Input: dimensioned drawing with shaded views. Units: mm. Origin: part minimum x, y, z. Give positions to 0.01 mm unless a question says otherwise; leave off trailing zeros. Loops run counter-clockwise (first coordinate to the right, second up) from the corner with the lowest first, then second, coordinate; pieces in that order, holes last.
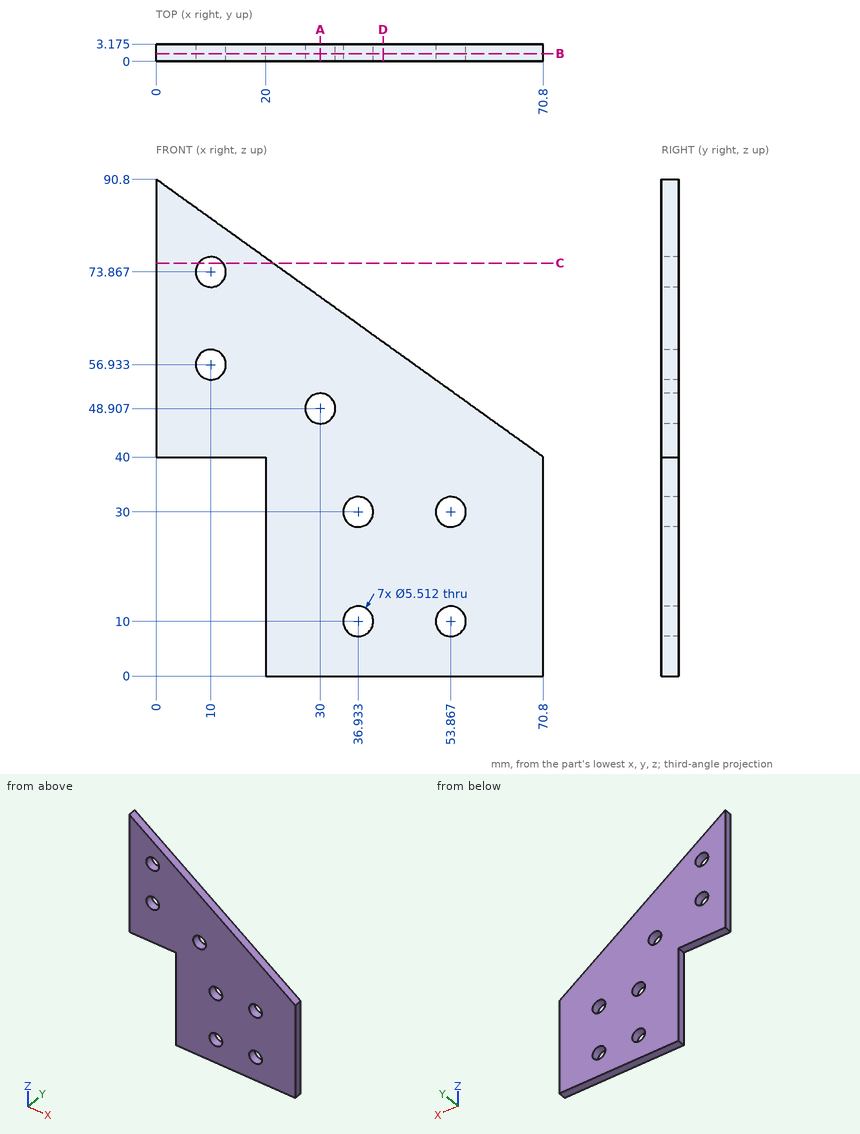
(1) Section A-A, the plane x = 30. Return the cut outline in (y, z) (1 decimal).
A:
outline: (0, 0) - (3.2, 0) - (3.2, 46.2) - (0, 46.2) - close; (0, 51.7) - (3.2, 51.7) - (3.2, 69.3) - (0, 69.3) - close
(2) Section B-B, the plane y = 1.4. Return the cut outline in (x, z), then the cut area to 3 significant figures.
A:
outline: (0, 40) - (20, 40) - (20, 0) - (70.8, 0) - (70.8, 40) - (0, 90.8) - close; hole circle Ø5.51 at (10, 56.93); hole circle Ø5.51 at (10, 73.87); hole circle Ø5.51 at (30, 48.91); hole circle Ø5.51 at (36.93, 10); hole circle Ø5.51 at (36.93, 30); hole circle Ø5.51 at (53.87, 10); hole circle Ø5.51 at (53.87, 30)
area: 3,660 mm2
(3) Section C-C, the plane z = 75.5. Return the cut outline in (x, y) (1 decimal).
A:
outline: (0, 0) - (7.8, 0) - (7.8, 3.2) - (0, 3.2) - close; (12.2, 0) - (21.3, 0) - (21.3, 3.2) - (12.2, 3.2) - close
(4) Ray query, line 1 along Z through (x, y) = (10, 2.7) (1 decimal); line 2 along X through (y, z) = (2, 28) (1 decimal); line 3 along Z through (x, y) = (34.5, 1.5) (1 decimal). Return the intervals inside material, ascending.
A:
line 1: z = 40 to 54.2, 59.7 to 71.1, 76.6 to 83.6
line 2: x = 20 to 35, 38.8 to 52, 55.8 to 70.8
line 3: z = 0 to 8.7, 11.3 to 28.7, 31.3 to 66
(5) Section D-D, the plane x = 41.5. Return the cut outline in (y, z) (1 decimal), then the cut area to 3 significant figures.
A:
outline: (0, 0) - (3.2, 0) - (3.2, 61) - (0, 61) - close
area: 194 mm2
(6) First-contact query: pin 1 (1 mm diameter, centred on x = 35, y = 2.5, fed in from +Z) (1 decimal); pin 2 (9 mm diameter, centred on x = 30, z = 48.91, fed in from +Y) (3 decimals); pin 3 (1 mm diameter, centred on x = 10.5, y = 2, fed in from +Z) (1 decimal); pin 4 (1.6 mm diameter, centred on x = 5.5, y = 1.5, fed in from -Z). Flat tips, straight axial feed; report the tip coordinate or a pass-through.
A:
pin 1: stops at z = 66
pin 2: stops at y = 3.175
pin 3: stops at z = 83.6
pin 4: stops at z = 40
